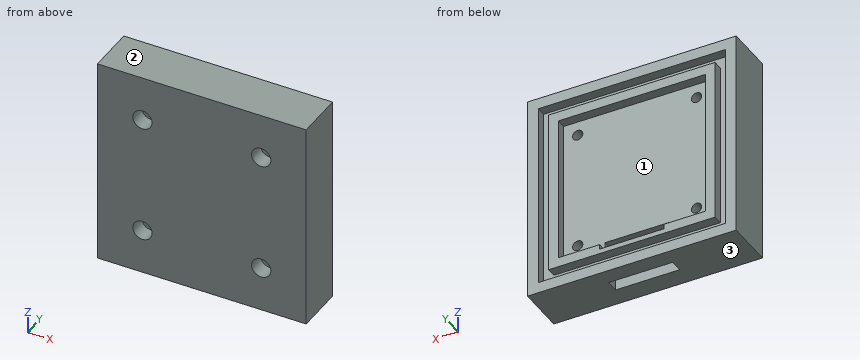
from build123d import *

# Parameters (mm, degrees)
SKETCH_1_W           = 65
SKETCH_1_H           = 65
EXTRUDE_1_DEPTH      = 15
SKETCH_2_R           = 1.6
CUT_EXTRUDE_1_DEPTH  = 16
SKETCH_3_W           = 45.8
SKETCH_3_H           = 45.8
CUT_EXTRUDE_2_DEPTH  = 3
SKETCH_4_W           = 58.2
SKETCH_4_H           = 58.2
SKETCH_4_W_2         = 51.8
SKETCH_4_H_2         = 51.8
CUT_EXTRUDE_3_DEPTH  = 3
SKETCH_7_R           = 3
CUT_EXTRUDE_6_DEPTH  = 5
SKETCH_10_W          = 20
SKETCH_10_H          = 4
CUT_EXTRUDE_9_DEPTH  = 9
SKETCH_11_W          = 20
SKETCH_11_H          = 4
CUT_EXTRUDE_10_DEPTH = 9
FILLET_2_R           = 4
FILLET_3_R           = 1


with BuildPart() as part:
    # 草图1 → 凸台-拉伸1 (new body)
    with BuildSketch(Plane(origin=(0, 0, 0), x_dir=(1, 0, 0), z_dir=(0, 1, 0))):
        with Locations((32.5, -32.5)):
            Rectangle(SKETCH_1_W, SKETCH_1_H)
    extrude(amount=EXTRUDE_1_DEPTH)

    # 草图2 → 切除-拉伸1 (cut, through all)
    with BuildSketch(Plane(origin=(0, 0, 0), x_dir=(-1, 0, 0), z_dir=(0, -1, 0))):
        with Locations((-14, -51)):
            Circle(SKETCH_2_R)
        with Locations((-51, -51)):
            Circle(SKETCH_2_R)
        with Locations((-14, -14)):
            Circle(SKETCH_2_R)
        with Locations((-51, -14)):
            Circle(SKETCH_2_R)
    extrude(amount=-CUT_EXTRUDE_1_DEPTH, mode=Mode.SUBTRACT)

    # 草图3 → 切除-拉伸2 (cut)
    with BuildSketch(Plane(origin=(0, 15, 0), x_dir=(1, 0, 0), z_dir=(0, 1, 0))):
        with Locations((32.5, -32.5)):
            Rectangle(SKETCH_3_W, SKETCH_3_H)
    extrude(amount=-CUT_EXTRUDE_2_DEPTH, mode=Mode.SUBTRACT)

    # 草图4 → 切除-拉伸3 (cut)
    with BuildSketch(Plane(origin=(0, 15, 0), x_dir=(1, 0, 0), z_dir=(0, 1, 0))):
        with Locations((32.5, -32.5)):
            Rectangle(SKETCH_4_W, SKETCH_4_H)
        with Locations((32.5, -32.5)):
            Rectangle(SKETCH_4_W_2, SKETCH_4_H_2, mode=Mode.SUBTRACT)
    extrude(amount=-CUT_EXTRUDE_3_DEPTH, mode=Mode.SUBTRACT)

    # 草图7 → 切除-拉伸6 (cut)
    with BuildSketch(Plane(origin=(0, 0, 0), x_dir=(-1, 0, 0), z_dir=(0, -1, 0))):
        with Locations((-14, -14)):
            Circle(SKETCH_7_R)
        with Locations((-14, -51)):
            Circle(SKETCH_7_R)
        with Locations((-51, -14)):
            Circle(SKETCH_7_R)
        with Locations((-51, -51)):
            Circle(SKETCH_7_R)
    extrude(amount=-CUT_EXTRUDE_6_DEPTH, mode=Mode.SUBTRACT)

    # 草图10 → 切除-拉伸9 (cut)
    with BuildSketch(Plane(origin=(0, 15, 0), x_dir=(1, 0, 0), z_dir=(0, 1, 0))):
        with Locations((32.5, -10.1)):
            Rectangle(SKETCH_10_W, SKETCH_10_H)
    extrude(amount=-CUT_EXTRUDE_9_DEPTH, mode=Mode.SUBTRACT)

    # 草图11 → 切除-拉伸10 (cut)
    with BuildSketch(Plane(origin=(0, 0, 0), x_dir=(-1, 0, 0), z_dir=(0, 0, -1))):
        with Locations((-32.5, 8)):
            Rectangle(SKETCH_11_W, SKETCH_11_H)
    extrude(amount=-CUT_EXTRUDE_10_DEPTH, mode=Mode.SUBTRACT)

    # 圆角2
    fillet_2_edges = [part.edges().sort_by_distance(p)[0] for p in [
        (32.5, 6, 12.1),
    ]]
    fillet(fillet_2_edges, radius=FILLET_2_R)

    # 圆角3
    fillet_3_edges = [part.edges().sort_by_distance(p)[0] for p in [
        (32.5, 10, 8.1),
    ]]
    fillet(fillet_3_edges, radius=FILLET_3_R)


solid = part.part
Check sheet for the modelled part. Datum: model origin and axes. Units: mm. Face numbers are marked on the shaded views. Give positions to 0.01 mm unless a question says otherwise; leave off trailing zeros. Loops run counter-clockwise (first coordinate to the right, second up) from the corner with the lowest first, then second, coordinate; pieces in that order, holes last. Notation, with made-up numbers: M 58.5,55.25 L 72.5,55.25 A29 ccw 72.5,89.25 Z; hole C 80.25,85 d3. An arc over 180 degrees is marked long. Answer as a JSON object with one key per item and string values. Group by question number.
Q1. Cross-section at D-D on x = 44.5. Record the cut outline in (y, z), then the cut area to 3 significant figures.
Q2. Cross-section at C-C on y = 4. Record the cut outline in (x, z).
Q3. Material ranges on line 1 along Z through (x, y) = (14, 13.75); line 2 along X through (y, z) = (13, 55.5); line 3 along X through (y, z) = (2.5, 14), recorded low to high. Write a range as [from, to].
Q4. Cross-section at A-A on z = 51. Give the number of separate pieces and of enclosed holes in the cut face, then the cut area to 3 significant figures.
Q5. Go/stop test with a flat-tipped pin: P1, Ø5.5, axis at x = 51, z = 14, coming from the +Y side. Record where the tip stops, or that it passes through.
Q6. Release check for a two-part mould opening along Z. For the marked faces 1, 2 and 3 record: released by +Z, released by -Z, zero draft, split by the parting line, or undercut.
Evaluation:
{
 "1": {"outline": "M 0,0 L 15,0 L 15,3.4 L 12,3.4 L 12,6.6 L 15,6.6 L 15,9.6 L 12,9.6 L 12,55.4 L 15,55.4 L 15,58.4 L 12,58.4 L 12,61.6 L 15,61.6 L 15,65 L 0,65 Z", "area": "818 mm2"},
 "2": {"outline": "M 0,0 L 65,0 L 65,65 L 0,65 Z; hole C 14,14 d6; hole C 14,51 d6; hole C 51,14 d6; hole C 51,51 d6"},
 "3": {"line 1": "z = [0, 3.4], [6.6, 9.6], [55.4, 58.4], [61.6, 65]", "line 2": "x = [0, 3.4], [6.6, 58.4], [61.6, 65]", "line 3": "x = [0, 11], [17, 48], [54, 65]"},
 "4": {"separate pieces": "3", "enclosed holes": "0", "area": "714 mm2"},
 "5": {"P1": "stops at y = 12"},
 "6": {"face 1": "undercut", "face 2": "released by +Z", "face 3": "released by -Z"}
}
